from build123d import *

# Parameters (mm, degrees)
BOSS_EXTRUDE1_DEPTH                = 2
F_1_16_0_0625_DIAMETER_HOLE2_D     = 1.5875
F_1_16_0_0625_DIAMETER_HOLE2_DEPTH = 19.05
F_1_16_0_0625_DIAMETER_HOLE2_TIP   = 0.476933116


with BuildPart() as part:
    # Sketch1 → Boss-Extrude1 (new body)
    with BuildSketch(Plane(origin=(0, 0, -49.2125), x_dir=(-1, 0, 0), z_dir=(0, 0, -1))):
        with BuildLine():
            Line((23.8125, 8.636), (-23.8125, 8.636))
            ThreePointArc((-23.8125, 8.636), (-26.237169153, 7.631669153), (-27.2415, 5.207))
            Line((-27.2415, 5.207), (-27.2415, -5.207))
            ThreePointArc((-27.2415, -5.207), (-26.237169153, -7.631669153), (-23.8125, -8.636))
            Line((-23.8125, -8.636), (23.8125, -8.636))
            ThreePointArc((23.8125, -8.636), (26.237169153, -7.631669153), (27.2415, -5.207))
            Line((27.2415, -5.207), (27.2415, 5.207))
            ThreePointArc((27.2415, 5.207), (26.237169153, 7.631669153), (23.8125, 8.636))
        make_face()
    extrude(amount=-BOSS_EXTRUDE1_DEPTH)

    # 1/16 (0.0625) Diameter Hole2
    with Locations(Plane(origin=(25.223, 0, -47.2125), x_dir=(1, 0, 0), z_dir=(0, 0, 1))):
        with Locations((0, 0), (-50.446, 0)):
            Hole(F_1_16_0_0625_DIAMETER_HOLE2_D / 2, depth=F_1_16_0_0625_DIAMETER_HOLE2_DEPTH)
            with Locations((0, 0, -(F_1_16_0_0625_DIAMETER_HOLE2_DEPTH + F_1_16_0_0625_DIAMETER_HOLE2_TIP / 2))):  # 118° drill point
                Cone(0, F_1_16_0_0625_DIAMETER_HOLE2_D / 2, F_1_16_0_0625_DIAMETER_HOLE2_TIP, mode=Mode.SUBTRACT)


solid = part.part
Model file for the job. Use its own axes, mm. Round coordinates to 2 decimals unless told otherwise and drop trailing zeros. Order: outer loops, then holes, each group sorted by start corner. A loop starts at its lowest first (then second) coordinate and runs counter-clockwise, first axis right, second up.
(1) Pull direction X, two halves, no side cores. Call faces 1 (the face through (0, -8.636, -48)), 2 (the face through (-25.98, 0.24, -48.23)), 3 (the face through (26.21, 7.66, -48.23)), 4 (the face through (-26.264, 7.605, -48.226)): released by +X, released by -X, zero draft, split by the parting line, or undercut.
(2) Band-saw the part on A-A (y = 0). List the corners of the cut face in (x, z), then the cut area to 3 significant figures.
(3) Drill centre lines: line 1 (X direction, y = -6.75, z = -47.8); line 2 (X direction, y = 6.5, z = -49). Where is each one in solid material? Low to high.
Verdict:
1. face 1: zero draft
1. face 2: undercut
1. face 3: released by +X
1. face 4: released by -X
2. outline: (-27.24, -49.21) - (-26.02, -49.21) - (-26.02, -47.21) - (-27.24, -47.21) - close; (-24.43, -49.21) - (24.43, -49.21) - (24.43, -47.21) - (-24.43, -47.21) - close; (26.02, -49.21) - (27.24, -49.21) - (27.24, -47.21) - (26.02, -47.21) - close
2. area: 103 mm2
3. line 1: x = -26.87 to 26.87
3. line 2: x = -26.99 to 26.99
